Geometry check sheet. Reference: drawing and pictorial views, mm from the part's lowest x, y, z. Round coordinates to 2 decimals unless told otherwise and drop trailing zeros. Order: outer loops, then holes, each group sorted by start corner. A loop starts at its lowest first (then second) coordinate and runs counter-clockwise, first axis right, second up.
(1) Sectioned sample at B-B (z = 55). Record the boundary of the cut face in (x, y).
(2) Material ranges on line 1 along X through (y, z) = (0.55, 5); line 2 along Z through (x, y) = (37.5, 0.65); line 3 along X through (y, z) = (0.75, 54), recorded low to high.
(3) Sectioned sample at A-A (x = 5). Record the boundary of the cut face in (y, z).
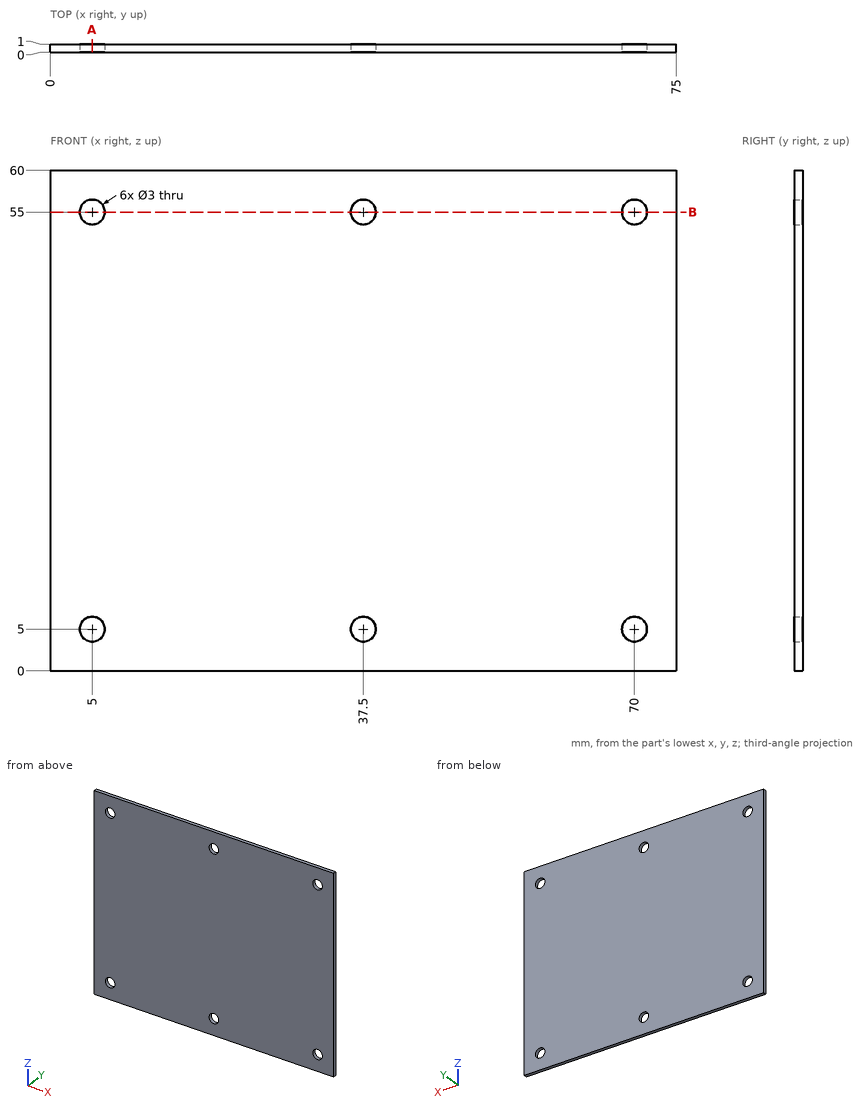
Answer below:
1. outline: (0, 0) - (3.5, 0) - (3.5, 1) - (0, 1) - close; (6.5, 0) - (36, 0) - (36, 1) - (6.5, 1) - close; (39, 0) - (68.5, 0) - (68.5, 1) - (39, 1) - close; (71.5, 0) - (75, 0) - (75, 1) - (71.5, 1) - close
2. line 1: x = 0 to 3.5, 6.5 to 36, 39 to 68.5, 71.5 to 75
2. line 2: z = 0 to 3.5, 6.5 to 53.5, 56.5 to 60
2. line 3: x = 0 to 3.88, 6.12 to 36.38, 38.62 to 68.88, 71.12 to 75
3. outline: (0, 0) - (1, 0) - (1, 3.5) - (0, 3.5) - close; (0, 6.5) - (1, 6.5) - (1, 53.5) - (0, 53.5) - close; (0, 56.5) - (1, 56.5) - (1, 60) - (0, 60) - close
